Source: three-view drawing plus pictorial views. Frame: mm from the lowest corner of the part. A direction names the side the tool comes from. Give positions to 0.01 mm unless a question says otherwise; leave off trailing zeros. Order: outer loops, then holes, each group sorted by start corner. A loop starts at its lowest first (then second) coordinate and runs counter-clockwise, first axis right, second up.
1) Access query for the marked faces 1 and 2. Directions: +Z, -Z, +X, -X, +Y, -Y. A direction counts if a zero-diameter tool reaches every point of the face in a straight line with its end or side. Return the directions, or none.
2) Section A-A, the plane y = 18.25. Return loops of the section in (x, z).
3) Section B-B, the plane x = 14.5. Return loops of the section in (y, z).
4) First-contact query: P1, Ø10, axis at x = 62.5, y = 18.5, coming from the -Z side; P2, Ø1.5, axis at y = 12, z = 2, coming from the -X side. Flat tips, straight axial feed; report the tip coordinate or a pass-through.
5) Material intervals for line 1 (X direction, y = 16.5, z = 0.35); line 2 (Z direction, x = 81, y = 12.75), sorted ascending.
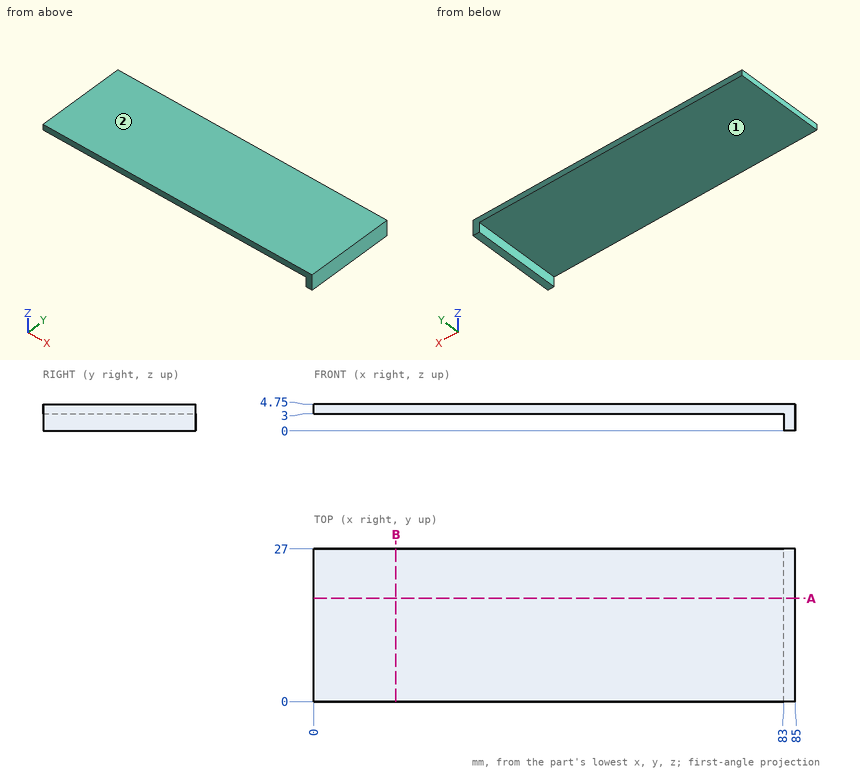
From the geometry:
1. face 1: -Z, -X, +Y, -Y
1. face 2: +Z, +X, -X, +Y, -Y
2. outline: (0, 3) - (83, 3) - (83, 0) - (85, 0) - (85, 4.75) - (0, 4.75) - close
3. outline: (0, 3) - (27, 3) - (27, 4.75) - (0, 4.75) - close
4. P1: stops at z = 3
4. P2: stops at x = 83
5. line 1: x = 83 to 85
5. line 2: z = 3 to 4.75
